Here's the drawing with two shaded views (mm, measured from the low corner). I have some questions. Give positions to 0.01 mm unless a question says otherwise; leave off trailing zeros. Write each loop counter-clockwise with the first axis right and the second up, starting at its lowest first coordinate (ties: lowest second). Pieces come first, ordered by that corner, then holes.
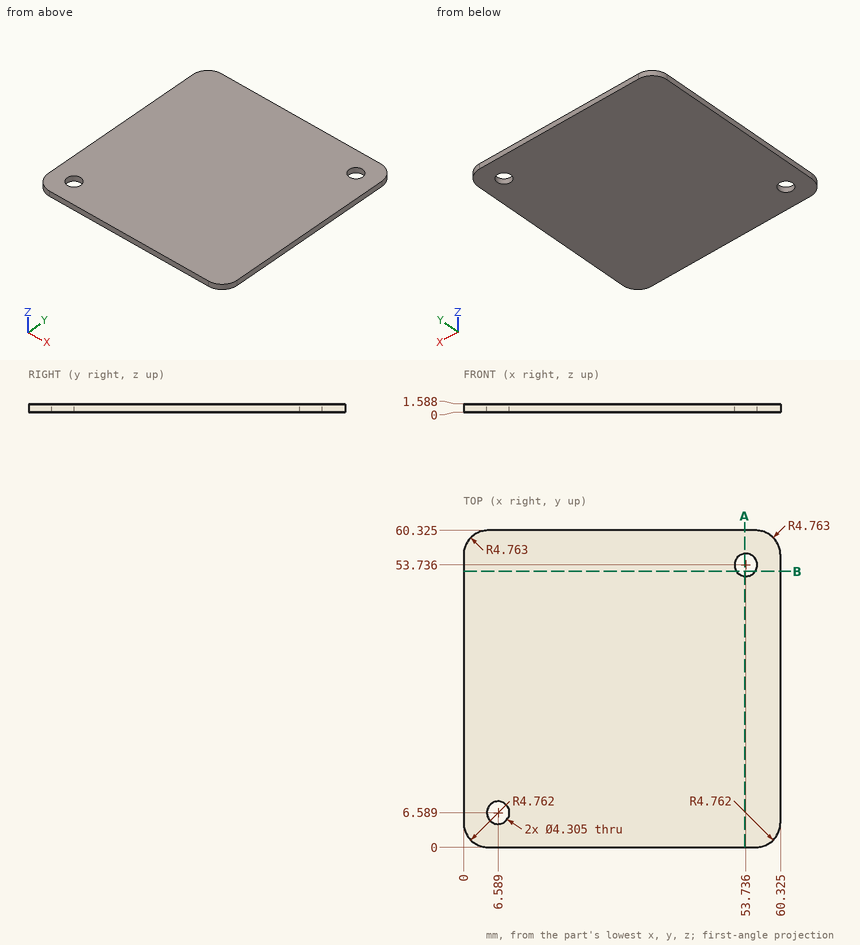
1) Please list where these lines run through material, in increasing order: L1, parallel to Y at x = 55.5, z = 0.95 (1 decimal); L2, parallel to X at y = 3, z = 1.3; L3, parallel to Y at x = 58.5, z = 1.3 (1 decimal).
Values follow:
L1: y = 0 to 52.5, 55 to 60.3
L2: x = 0.34 to 59.99
L3: y = 1 to 59.3
2) Suppose I cut it at A-A on x = 53.5. Write out the boundary of the cut face in (y, z) (1 decimal).
Values follow:
outline: (0, 0) - (51.6, 0) - (51.6, 1.6) - (0, 1.6) - close; (55.9, 0) - (60.3, 0) - (60.3, 1.6) - (55.9, 1.6) - close
3) For pin 1 Ø5.5 at (x, y) = (53.74, 53.74) entering from -Z, with a flat end and sliding along its axis, tell me the tip position at first contact or that it passes through.
Values follow:
pin 1: stops at z = 0
4) Suppose I cut it at B-B on y = 52.5. Write out the boundary of the cut face in (x, z) (1 decimal).
Values follow:
outline: (0, 0) - (52, 0) - (52, 1.6) - (0, 1.6) - close; (55.5, 0) - (60.3, 0) - (60.3, 1.6) - (55.5, 1.6) - close
